Work out the finished part from the listing and answer in its coordinate system (mm). A direction names the side the tool comes from. Coordinates: 2 decimals unless noted, no trailing zeros. Order: outer loops, then holes, each group sorted by start corner. A loop starts at its lowest first (then second) coordinate and runs counter-clockwise, first axis right, second up. Notation, with made-up numbers: (71.25, -4) -> (101.25, -4) arc R24 cw to (101.25, 18) -> close; hole circle Ø11 at (4.25, -6.75). An arc over 180 degrees is marked (long way). Answer as CSV lines item,"result". Start each with the question number.
Item 1: Each of these flat-tipped pins is pushed along its axis until it touches: pin 1 Ø3 at (x, z) = (2.5, -7.5) entering from -Y; pin 2 Ø2 at (x, y) = (6.5, 6) entering from -Z; pin 3 Ø2 at (x, y) = (2, -9) entering from +Z. Where does it stop, or does it pass through?
Item 2: Which of the six approach directions +Z, -Z, +X, -X, +Y, -Y give full straight-line access (tool end or side, diameter ignored) to faces 4 (the face through (4.93, 9.306, -5.38)), 5 (the face through (4.93, 0.809, -11.874)), 6 (the face through (4.93, 11.26, 3.855)), 7 (the face through (4.93, -11.9, 0.82))?
Item 3: Section C-C (z = 11.25) is taken. Write down the section's boundary in (x, y).
Item 4: For a pull along Z with two mould halves and no side action, classify faces 1 (the face through (4.93, 5.37, -9.31)), 2 (the face through (4.93, -3.855, 11.26)), 3 (the face through (0, -3, 3)) as pulls with the +Z half, pulls with the -Z half, needs draft (parallel to the pull), parting line crosses it, or undercut.
Item 5: Section A-A (y = 0) is taken. Write down the section's boundary in (x, z), then the cut area to 3 significant figures.
Item 6: Straight lines are drawn through the part: L1, parallel to Y at x = 6.75, z = 0; L2, parallel to Y at x = 4.25, z = -9.75; L3, parallel to Y at x = 9.25, z = -11. For each, find the intervals that lie inside material, in ascending order.
```python
from build123d import *

# Parameters (mm, degrees)
BASPROSKE_W        = 10
BASPROSKE_H        = 13
TOOTHCUT_DEPTH     = 21.928449536
TEETHCUTS_COUNT    = 24
TEETHCUTS_ANGLE    = 345
BORSKE_R           = 2.5
BORE_DEPTH         = 50.0000508
SKETCH1_R          = 3
CUT_EXTRUDE1_DEPTH = 21.83151436


with BuildPart() as part:
    # BasProSke → Base-Revolve (revolve)
    with BuildSketch(Plane(origin=(0, 0, 0), x_dir=(1, 0, 0), z_dir=(0, 1, 0)), mode=Mode.PRIVATE) as base_revolve_sk:
        with Locations((5, 6.5)):
            Rectangle(BASPROSKE_W, BASPROSKE_H)
    revolve(base_revolve_sk.sketch.rotate(Axis((-10, 0, 0), (1, 0, 0)), 180), axis=Axis((-10, 0, 0), (1, 0, 0)))

    # TooCutSke → ToothCut (cut, through all)
    with BuildSketch(Plane(origin=(0, 0, 0), x_dir=(0, 0, -1), z_dir=(1, 0, 0))):
        with BuildLine():
            ThreePointArc((0.483448384, 10.738122679), (0, 10.749), (-0.483448384, 10.738122679))
            ThreePointArc((-0.483448384, 10.738122679), (-0.821636462, 11.902754369), (-1.44092227, 12.945454344))
            ThreePointArc((-1.44092227, 12.945454344), (0, 13.0254), (1.44092227, 12.945454344))
            ThreePointArc((1.44092227, 12.945454344), (0.821636462, 11.902754369), (0.483448384, 10.738122679))
        make_face()
    toothcut = extrude(amount=TOOTHCUT_DEPTH, mode=Mode.SUBTRACT)

    # TeethCuts: ToothCut ×24 about axis
    teethcuts_axis = Axis((-10, 0, 0), (1, 0, 0))
    for i in range(1, TEETHCUTS_COUNT):
        add(toothcut.rotate(teethcuts_axis, i * TEETHCUTS_ANGLE / (TEETHCUTS_COUNT - 1)), mode=Mode.SUBTRACT)

    # BorSke → Bore (cut, symmetric)
    with BuildSketch(Plane(origin=(0, 0, 0), x_dir=(0, 0, -1), z_dir=(1, 0, 0))):
        with Locations(Location((0, 0, 0), (0, 0, 180))):
            Circle(BORSKE_R)
    extrude(amount=BORE_DEPTH, both=True, mode=Mode.SUBTRACT)

    # Sketch1 → Cut-Extrude1 (cut, through all)
    with BuildSketch(Plane(origin=(10, 0, 0), x_dir=(0, 0, -1), z_dir=(1, 0, 0))):
        Circle(SKETCH1_R)
    extrude(amount=-CUT_EXTRUDE1_DEPTH, mode=Mode.SUBTRACT)


solid = part.part
```
Checked values:
1,pin 1,"stops at y = -10.48"
1,pin 2,"stops at z = -12"
1,pin 3,"stops at z = 10.25"
2,face 4,"+X, -X"
2,face 5,"-Z, +X, -X"
2,face 6,"+X, -X, +Y"
2,face 7,"+X, -X, -Y"
3,outline,"(0, -5.27) -> (10, -5.27) -> (10, -3.85) -> (0, -3.85) -> close; (0, -2.33) -> (10, -2.33) -> (10, -0.59) -> (0, -0.59) -> close; (0, 0.59) -> (10, 0.59) -> (10, 2.33) -> (0, 2.33) -> close; (0, 3.85) -> (10, 3.85) -> (10, 5.27) -> (0, 5.27) -> close"
4,face 1,"undercut"
4,face 2,"pulls with the +Z half"
4,face 3,"needs draft"
5,outline,"(0, -10.75) -> (10, -10.75) -> (10, -3) -> (0, -3) -> close; (0, 3) -> (10, 3) -> (10, 10.75) -> (0, 10.75) -> close"
5,area,"155 mm^2"
6,L1,"y = -10.75 to -3, 3 to 10.75"
6,L2,"y = -8.06 to -6.47, -5.03 to 5.03, 6.47 to 8.06"
6,L3,"y = -5.26 to -3.66, -2.34 to -0.53, 0.53 to 2.34, 3.66 to 5.26"
